Build history of the part. All positions in model axes, mm. A direction names the side the tool comes from. Round coordinates to 2 decimals unless told otherwise and drop trailing zeros. Write each loop counter-clockwise with the first axis right and the second up, starting at its lowest first coordinate (ties: lowest second). Pieces come first, ordered by that corner, then holes.
from build123d import *

# Parameters (mm, degrees)
SKETCH009_R     = 21
PAD002_DEPTH    = 6
SKETCH010_R     = 4
PAD003_DEPTH    = 6
SKETCH011_R     = 1.65
POCKET007_DEPTH = 6.001
SKETCH012_R     = 9.05
POCKET008_DEPTH = 4
SKETCH013_R     = 8.05
POCKET009_DEPTH = 6.001


with BuildPart() as part:
    # Sketch009 → Pad002 (new body)
    with BuildSketch(Plane.XY):
        Circle(SKETCH009_R)
    extrude(amount=PAD002_DEPTH)

    # Sketch010 (on DatumPlane) → Pad003 (join)
    with BuildSketch(Plane.XY.offset(6)):
        with Locations((-12.727922, 12.727922)):
            Circle(SKETCH010_R)
        with Locations((0, 18)):
            Circle(SKETCH010_R)
        with Locations((12.727922, 12.727922)):
            Circle(SKETCH010_R)
        with Locations((15.588457, -9)):
            Circle(SKETCH010_R)
        with Locations((-15.588457, -9)):
            Circle(SKETCH010_R)
        with Locations((0, -18)):
            Circle(SKETCH010_R)
    extrude(amount=-PAD003_DEPTH)

    # Sketch011 (on DatumPlane) → Pocket007 (cut, through all)
    with BuildSketch(Plane.XY.offset(6)):
        with Locations((-12.727922, 12.727922)):
            Circle(SKETCH011_R)
        with Locations((0, 18)):
            Circle(SKETCH011_R)
        with Locations((12.727922, 12.727922)):
            Circle(SKETCH011_R)
        with Locations((-15.588457, -9)):
            Circle(SKETCH011_R)
        with Locations((15.588457, -9)):
            Circle(SKETCH011_R)
        with Locations((0, -18)):
            Circle(SKETCH011_R)
    extrude(amount=-POCKET007_DEPTH, mode=Mode.SUBTRACT)

    # Sketch012 (on DatumPlane) → Pocket008 (cut)
    with BuildSketch(Plane.XY.offset(6)):
        Circle(SKETCH012_R)
    extrude(amount=-POCKET008_DEPTH, mode=Mode.SUBTRACT)

    # Sketch013 (on DatumPlane) → Pocket009 (cut, through all)
    with BuildSketch(Plane.XY.offset(6)):
        Circle(SKETCH013_R)
    extrude(amount=-POCKET009_DEPTH, mode=Mode.SUBTRACT)


with BuildPart() as part_1:
    # Body001 placement: moved
    add(part.part.moved(Location((0, 0, 14))))


solid = part_1.part
1) Slice it at D-D (z = 17.6). Write the cut outline in (x, y), plus the area to 3 significant figures.
Results:
outline: (-19.44, -7.93) arc R4 ccw to (-16.59, -12.87) arc R21 ccw to (-2.85, -20.81) arc R4 ccw to (2.85, -20.81) arc R21 ccw to (16.59, -12.87) arc R4 ccw to (19.44, -7.93) arc R21 ccw to (16.73, 12.7) arc R4 ccw to (12.7, 16.73) arc R21 ccw to (2.85, 20.81) arc R4 ccw to (-2.85, 20.81) arc R21 ccw to (-12.7, 16.73) arc R4 ccw to (-16.73, 12.7) arc R21 ccw to start; hole circle Ø3.3 at (-15.59, -9); hole circle Ø3.3 at (-12.73, 12.73); hole circle Ø18.1 at (0, 0); hole circle Ø3.3 at (0, -18); hole circle Ø3.3 at (0, 18); hole circle Ø3.3 at (12.73, 12.73); hole circle Ø3.3 at (15.59, -9)
area: 1,100 mm2
2) Slice it at A-A (y = 0). Write the cut outline in (x, z), plus the area to 3 significant figures.
Results:
outline: (-21, 14) - (-8.05, 14) - (-8.05, 16) - (-9.05, 16) - (-9.05, 20) - (-21, 20) - close; (8.05, 14) - (21, 14) - (21, 20) - (9.05, 20) - (9.05, 16) - (8.05, 16) - close
area: 147 mm2
3) Pin check, flat tips, straight feed: pin 1 Ø2 at (x, z) = (-14.5, 19) entering from -Y; pin 2 Ø1.5 at (x, z) = (-2.5, 19) entering from +Y; pin 3 Ø3 at (x, z) = (6, 15) entering from +Y. Stop position of each tip, or through.
Results:
pin 1: stops at y = -16.09
pin 2: stops at y = 21.6
pin 3: stops at y = 20.51
4) Mould opens along Y. For faces 1 (the cylindrical face through (14.252, 12.096, 17.042)), 2 (the flat face through (9, 0, 14)), 3 (the cylindrical face through (0, 22, 17)) say: released by +Y, released by -Y, zero draft, split by the parting line, or undercut.
Results:
face 1: undercut
face 2: zero draft
face 3: released by +Y
5) Slice it at B-B (x = 0). Write the cut outline in (y, z), plus the area to 3 significant figures.
Results:
outline: (-22, 14) - (-19.65, 14) - (-19.65, 20) - (-22, 20) - close; (-16.35, 14) - (-8.05, 14) - (-8.05, 16) - (-9.05, 16) - (-9.05, 20) - (-16.35, 20) - close; (8.05, 14) - (16.35, 14) - (16.35, 20) - (9.05, 20) - (9.05, 16) - (8.05, 16) - close; (19.65, 14) - (22, 14) - (22, 20) - (19.65, 20) - close
area: 120 mm2
6) Which spindle directions (+Z, -Z, +X, -X, +Y, -Y) get a long thin tool onto all of the face, cutting with end or side? Do faces 4 (the cylindrical face through (-19.075, -10.961, 17.042)), 5 (the cylindrical face through (8.63, 2.72, 18.03)). Say none if no direction does.
Results:
face 4: +Z, -Z, -X
face 5: +Z
7) Slice it at C-C (x = 12). Write the cut outline in (y, z), plus the area to 3 significant figures.
Results:
outline: (-17.23, 14) - (11.25, 14) - (11.25, 20) - (-17.23, 20) - close; (14.21, 14) - (17.23, 14) - (17.23, 20) - (14.21, 20) - close
area: 189 mm2
8) Wall check: L1, parallel to Y at x = 0, z = 19; L2, parallel to Y at x = -15, z = 15.85; L3, parallel to X at y = -2.5, z = 17.95. Give the ranges that are in metal, low to high.
Results:
L1: y = -22 to -19.65, -16.35 to -9.05, 9.05 to 16.35, 19.65 to 22
L2: y = -14.7 to -10.54, -7.46 to 16.02
L3: x = -20.85 to -8.7, 8.7 to 20.85
